Autodesk Inventor part; units mm, degrees
ref_plane "YZ Plane" through (0, 0, 0) normal (1, 0, 0) x (0, 1, 0)
ref_plane "XZ Plane" through (0, 0, 0) normal (0, 1, 0) x (-1, 0, 0)
ref_plane "XY Plane" through (0, 0, 0) normal (0, 0, 1) x (1, 0, 0)
sketch "Sketch1" plane through (0, 0, 0) normal (0, 1, 0) x (-1, 0, 0)
  circle A0 centre (0, 0) radius 7.2
  dimension "d0" = 14.4
extrude "Extrusion1" add sketch "Sketch1" along normal blind 4
hole "Hole1" at (0, 0, 0) direction (0, 1, 0) diameter 4.9 end through all
hole "Hole2" at (0, 0, 0) direction (0, 1, 0) diameter 9.5 depth 3.1
hole "Hole3" at (0, 0, 0) direction (0, 1, 0) diameter 10 depth 1
properties part number "Hitec HS-5245MG gear 5 _2"
Can you work these out from the model? Positions are in its coordinate system, mm. A direction names the side the tool comes from. Coordinates: 2 decimals unless noted, no trailing zeros. Loops run counter-clockwise (first coordinate to the right, second up) from the corner with the lowest first, then second, coordinate; pieces in that order, holes last. Notation, with made-up numbers: M 9,4.25 L 32,4.25 A7 ccw 32,17.25 Z; hole C 39,35.25 d1. An arc over 180 degrees is marked long. Return JSON: item names as keys, results as strings. Group by question number.
Item 1: If I drill on L1, parallel to Z at x = 0, y = 2.3; L2, parallel to Z at x = 0, y = 0.75; L3, parallel to Y at x = 3.25, z = -2.75, over which ranges is the centre line in solid material (lowest first)? Write a range as from..to.
Item 2: Thinking about a two-plate mould opening in X: for faces 1 (the cylindrical face through (-6.87, 1.97, -2.16)), 2 (the cylindrical face through (4.88, 0.51, 1.08)), 3 (the flat face through (0, 4, -3)), which applies, released by +X, released by -X, zero draft, split by the parting line, or undercut?
Item 3: Imagine slicing it at C-C (x = 3.75). Please give me the cut outline in (y, z).
Item 4: On a 3-axis mill with a long thin cutter (end or side, diameter ignored), from which of +Z, -Z, +X, -X, +Y, -Y can I reach the whole of each face in a straight line? I mean faces 4 (the cylindrical face through (2.4, 3.6, 0.5)), 5 (the cylindrical face through (4.214, 2.065, -2.192)). Say none if no direction works.
Item 5: I'm going to push flat-ended pins straight in: pin 1 Ø7.5 at (x, z) = (0, 0) entering from -Y; pin 2 Ø1 at (y, z) = (1.5, -4.5) entering from -X. Where does each tip first touch, or does it pass through?
Item 6: Imagine slicing it at B-B (z = 0). Please give me the cut outline in (x, y), and give its area (3 significant figures).
Item 7: Imagine slicing it at D-D (y = 1.95). Please give me the cut outline in (x, z), and give its area (3 significant figures).
Item 8: Imagine slicing it at A-A (x = 0). Please give me the cut outline in (y, z), and give its area (3 significant figures).
Verdict:
{
 "1": {"L1": "z = -7.2..-4.75, 4.75..7.2", "L2": "z = -7.2..-5, 5..7.2", "L3": "y = 3.1..4"},
 "2": {"face 1": "split by the parting line", "face 2": "undercut", "face 3": "zero draft"},
 "3": {"outline": "M 0,-6.15 L 4,-6.15 L 4,6.15 L 0,6.15 L 0,3.31 L 1,3.31 L 1,2.92 L 3.1,2.92 L 3.1,-2.92 L 1,-2.92 L 1,-3.31 L 0,-3.31 Z"},
 "4": {"face 4": "+Y, -Y", "face 5": "-Y"},
 "5": {"pin 1": "stops at y = 3.1", "pin 2": "stops at x = -5.99"},
 "6": {"outline": "M -7.2,0 L -5,0 L -5,1 L -4.75,1 L -4.75,3.1 L -2.45,3.1 L -2.45,4 L -7.2,4 Z; M 2.45,3.1 L 4.75,3.1 L 4.75,1 L 5,1 L 5,0 L 7.2,0 L 7.2,4 L 2.45,4 Z", "area": "23.2 mm^2"},
 "7": {"outline": "C 0,0 d14.4; hole C 0,0 d9.5", "area": "92.0 mm^2"},
 "8": {"outline": "M 0,-7.2 L 4,-7.2 L 4,-2.45 L 3.1,-2.45 L 3.1,-4.75 L 1,-4.75 L 1,-5 L 0,-5 Z; M 0,5 L 1,5 L 1,4.75 L 3.1,4.75 L 3.1,2.45 L 4,2.45 L 4,7.2 L 0,7.2 Z", "area": "23.2 mm^2"}
}
